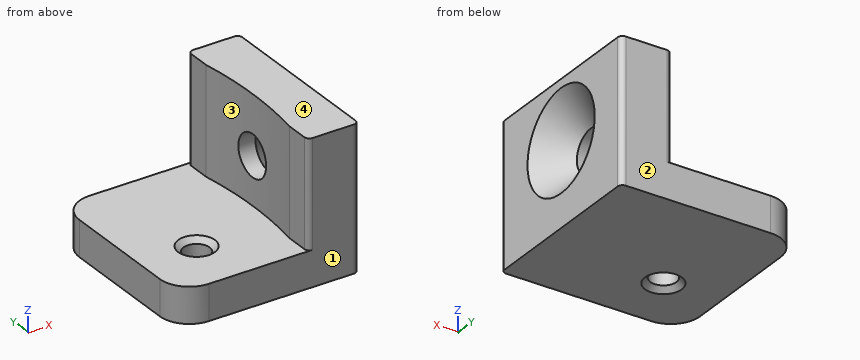
```python
from build123d import *

# Parameters (mm, degrees)
BOSS_EXTRUDE1_DEPTH                             = 9.271
CUT_EXTRUDE1_DEPTH                              = 24.491224021
CSK_FOR_M4_FLAT_HEAD_MACHINE_SCREW1_D           = 4.3
CSK_FOR_M4_FLAT_HEAD_MACHINE_SCREW1_CSINK_D     = 10.416
CSK_FOR_M4_FLAT_HEAD_MACHINE_SCREW1_CSINK_ANGLE = 90
FILLET2_R                                       = 3.048
FILLET3_R                                       = 0.508


with BuildPart() as part:
    # Sketch1 → Boss-Extrude1 (new, symmetric)
    with BuildSketch(Plane(origin=(0, 0, 0), x_dir=(1, 0, 0), z_dir=(0, 1, 0))):
        Polygon((-18.542, 4.953), (-7.62, 4.953), (-7.62, -6.096), (0, -6.096), (0, 8.636), (-18.542, 8.636), align=None)
    extrude(amount=BOSS_EXTRUDE1_DEPTH, both=True)

    # Sketch2 → Cut-Extrude1 (cut, through all)
    with BuildSketch(Plane(origin=(0, 0, -4.953), x_dir=(-1, 0, 0), z_dir=(0, 0, -1))):
        with BuildLine():
            Line((5.2832, 6.46179195), (5.2832, 15.24))
            Line((5.2832, 15.24), (52.002170663, 15.24))
            Line((52.002170663, 15.24), (52.002170663, -15.24))
            Line((52.002170663, -15.24), (5.2832, -15.24))
            Line((5.2832, -15.24), (5.2832, -6.46179195))
            ThreePointArc((5.2832, -6.46179195), (4.7752, 0), (5.2832, 6.46179195))
        make_face()
    extrude(amount=-CUT_EXTRUDE1_DEPTH, mode=Mode.SUBTRACT)

    # CSK for M4 Flat Head Machine Screw1 (through all)
    with Locations(Plane(origin=(0, 0, 0), x_dir=(0, 0, -1), z_dir=(1, 0, 0))):
        with Locations((0, 0)):
            CounterSinkHole(CSK_FOR_M4_FLAT_HEAD_MACHINE_SCREW1_D / 2, CSK_FOR_M4_FLAT_HEAD_MACHINE_SCREW1_CSINK_D / 2, counter_sink_angle=CSK_FOR_M4_FLAT_HEAD_MACHINE_SCREW1_CSINK_ANGLE)

    # Sketch5 → #6-32 Tapped Hole1 (revolve, cut)
    with BuildSketch(Plane(origin=(-12.7, -3.175, -8.636), x_dir=(0, 1, 0), z_dir=(1, 0, 0))):
        Polygon((0, 0), (0, 3.683), (1.905, 3.683), (1.35255, 3.13055), (1.35255, 0.55245), (1.905, 0), align=None)
    revolve(axis=Axis((-12.7, -3.175, -14.986), (0, 0, 1)), mode=Mode.SUBTRACT)

    # Fillet2
    fillet2_edges = [part.edges().sort_by_distance(p)[0] for p in [
        (-18.542, 9.271, -6.7945),
        (-18.542, -9.271, -6.7945),
    ]]
    fillet(fillet2_edges, radius=FILLET2_R)

    # Fillet3
    fillet3_edges = [part.edges().sort_by_distance(p)[0] for p in [
        (-5.2832, -9.271, 0.5715),
        (-5.2832, 9.271, 0.5715),
        (0, 9.271, -1.27),
        (0, -9.271, -1.27),
    ]]
    fillet(fillet3_edges, radius=FILLET3_R)


solid = part.part
```
Here's how the part is built. I have some questions about the finished solid (model axes, mm). Face numbers are marked on the shaded views. Round coordinates to 2 decimals unless told otherwise and drop trailing zeros. Loops run counter-clockwise (first coordinate to the right, second up) from the corner with the lowest first, then second, coordinate; pieces in that order, holes last.
1. Thinking about a two-plate mould opening in Y: for the marked faces 1, 2, 3 and 4, which applies, released by +Y, released by -Y, zero draft, split by the parting line, or undercut?
Answers:
face 1: released by -Y
face 2: released by +Y
face 3: undercut
face 4: zero draft
2. If I drill on probe 1 along Y at (x, z) = (-12.7, -6.3); probe 2 along Y at (x, z) = (-3.9, 0); probe 3 along Z at (x, y) = (-3.75, 0), over which ranges is the centre line in solid material (lowest first)?
Answers:
probe 1: y = -9.27 to -4.53, -1.82 to 9.27
probe 2: y = -9.27 to -2.15, 2.15 to 9.27
probe 3: z = -8.64 to -2.15, 2.15 to 6.1
3. Suppose I cut it at C-C, the plane z = 0. Please give me the cut outline in (x, y), and give its area (3 significant figures).
Answers:
outline: (-5.28, -8.76) arc R0.51 ccw to (-4.78, -9.27) - (-0.51, -9.27) arc R0.51 ccw to (0, -8.76) - (0, -5.21) - (-3.06, -2.15) - (-4.83, -2.15) arc R41.35 cw to (-5.28, -6.46) - close; (-5.28, 6.46) arc R41.35 cw to (-4.83, 2.15) - (-3.06, 2.15) - (0, 5.21) - (0, 8.76) arc R0.51 ccw to (-0.51, 9.27) - (-4.78, 9.27) arc R0.51 ccw to (-5.28, 8.76) - close
area: 63.4 mm2
4. Suppose I cut it at B-B, the plane y = 0. Please give me the cut outline in (x, z).
Answers:
outline: (-18.54, -8.64) - (0, -8.64) - (0, -5.21) - (-3.06, -2.15) - (-4.78, -2.15) - (-4.78, -4.95) - (-18.54, -4.95) - close; (-4.78, 2.15) - (-3.06, 2.15) - (0, 5.21) - (0, 6.1) - (-4.78, 6.1) - close
5. Suppose I cut it at D-D, the plane y = -5.5. Please give me the cut outline in (x, z), and give its area (3 significant figures).
Answers:
outline: (-18.54, -8.64) - (0, -8.64) - (0, 6.1) - (-5.14, 6.1) - (-5.14, -4.95) - (-18.54, -4.95) - close
area: 125 mm2
6. Will these pins go through, and if not, where does the flat tip stop? pin 1 (1.2 mm diameter, centred on y = 8, z = -0.5, fed in from -X); pin 2 (7 mm diameter, centred on x = -12.5, y = -3.5, fed in from +Z).
Answers:
pin 1: stops at x = -5.28
pin 2: stops at z = -4.95
7. Suppose I cut it at A-A, the plane x = -12.7. Please give me the cut outline in (y, z).
Answers:
outline: (-9.27, -8.64) - (-5.08, -8.64) - (-4.53, -8.08) - (-4.53, -5.51) - (-5.08, -4.95) - (-9.27, -4.95) - close; (-1.82, -8.08) - (-1.27, -8.64) - (9.27, -8.64) - (9.27, -4.95) - (-1.27, -4.95) - (-1.82, -5.51) - close
